Input: part model. Units: mm. Frame: model coordinates. Give positions to 0.01 mm unless a question says otherwise; leave off trailing zeros. Loops run counter-clockwise (first coordinate to the right, second up) from the corner with the lowest first, then second, coordinate; pieces in that order, holes last. Notation, with made-up numbers: M 37.25,-17 L 89.25,-17 A10 ccw 89.25,-7 Z; hole C 0.5,-18.5 d4. An arc over 180 degrees is marked long. Answer as a JSON object with one key per item and string values. Group by question number.
```python
from build123d import *

# Parameters (mm, degrees)
F0_W     = 127
F0_H     = 33.9515097439
F1_DEPTH = 35.56
F2_R     = 5.5188922036
F3_SIZE  = 5.08
F5_D     = 6.35
F6_R     = 5.08
F7_SIZE  = 5.08


with BuildPart() as f1:
    # F0 (on Top) → F1 (new body)
    with BuildSketch(Plane.XY):
        with Locations((63.5, -16.975754872)):
            Rectangle(F0_W, F0_H)
    extrude(amount=F1_DEPTH)

    # F2
    f2_edges = [f1.edges().sort_by_distance(p)[0] for p in [
        (0, -33.95151, 17.78),
    ]]
    fillet(f2_edges, radius=F2_R)

    # F3
    f3_edges = [f1.edges().sort_by_distance(p)[0] for p in [
        (127, -33.95151, 17.78),
    ]]
    chamfer(f3_edges, length=F3_SIZE)

    # F5 (through all)
    with Locations(Plane.XY.offset(35.56)):
        with Locations((27.8624333441, -11.6866370663)):
            Hole(F5_D / 2)

    # F6
    f6_edges = [f1.edges().sort_by_distance(p)[0] for p in [
        (121.92, -33.95151, 17.78),
    ]]
    fillet(f6_edges, radius=F6_R)

    # F7
    f7_edges = [f1.edges().sort_by_distance(p)[0] for p in [
        (127, 0, 17.78),
    ]]
    chamfer(f7_edges, length=F7_SIZE)


solid = f1.part
```
1. Section A-A (y = -10.5). Output: boundary loops of the cut face in (x, z).
2. Section C-C (y = -2.5). Output: boundary loops of the cut face in (x, z).
3. Section B-B (x = 26). Output: boundary loops of the cut face in (y, z), then the cut area to 3 significant figures.
4. Material intervals for L1, parallel to X at y = -12, z = 21.5; L2, parallel to X at y = -14.5, z = 21; L3, parallel to X at y = -29.5, z = 21, sorted ascending.
Geometry results:
{
 "1": {"outline": "M 0,0 L 24.92,0 L 24.92,35.56 L 0,35.56 Z; M 30.81,0 L 127,0 L 127,35.56 L 30.81,35.56 Z"},
 "2": {"outline": "M 0,0 L 124.42,0 L 124.42,35.56 L 0,35.56 Z"},
 "3": {"outline": "M -33.95,0 L -14.26,0 L -14.26,35.56 L -33.95,35.56 Z; M -9.12,0 L 0,0 L 0,35.56 L -9.12,35.56 Z", "area": "1,020 mm2"},
 "4": {"L1": "0 to 24.7, 31.02 to 127", "L2": "0 to 26.39, 29.33 to 127", "L3": "0.1 to 126.37"}
}
